```python
from build123d import *

# Parameters (mm, degrees)
SKETCH1_W           = 100
SKETCH1_H           = 300
SKETCH1_W_2         = 88
SKETCH1_H_2         = 91
SKETCH1_H_3         = 94
BOSS_EXTRUDE1_DEPTH = 6
SKETCH2_R           = 1.5
CUT_EXTRUDE1_DEPTH  = 6


with BuildPart() as part:
    # Sketch1 → Boss-Extrude1 (new body)
    with BuildSketch(Plane.XY):
        Rectangle(SKETCH1_W, SKETCH1_H)
        with Locations((0, 98.5)):
            Rectangle(SKETCH1_W_2, SKETCH1_H_2, mode=Mode.SUBTRACT)
        with Locations((0, -98.5)):
            Rectangle(SKETCH1_W_2, SKETCH1_H_2, mode=Mode.SUBTRACT)
        Rectangle(SKETCH1_W_2, SKETCH1_H_3, mode=Mode.SUBTRACT)
    extrude(amount=BOSS_EXTRUDE1_DEPTH)

    # Sketch2 → Cut-Extrude1 (cut)
    with BuildSketch(Plane.XY.offset(6)):
        with Locations((-47, 147)):
            Circle(SKETCH2_R)
        with Locations((47, 147)):
            Circle(SKETCH2_R)
        with Locations((47, 49)):
            Circle(SKETCH2_R)
        with Locations((47, -49)):
            Circle(SKETCH2_R)
        with Locations((47, -147)):
            Circle(SKETCH2_R)
        with Locations((-47, 49)):
            Circle(SKETCH2_R)
        with Locations((-47, -49)):
            Circle(SKETCH2_R)
        with Locations((-47, -147)):
            Circle(SKETCH2_R)
    extrude(amount=-CUT_EXTRUDE1_DEPTH, mode=Mode.SUBTRACT)


solid = part.part
```
CAD build for the part. Positions are in the model's coordinates, mm. A direction names the side the tool comes from. Round coordinates to 2 decimals unless told otherwise and drop trailing zeros. Write each loop counter-clockwise with the first axis right and the second up, starting at its lowest first coordinate (ties: lowest second). Pieces come first, ordered by that corner, then holes. Notation, with made-up numbers: (14.5, 77.25) - (24.5, 77.25) arc R21 cw to (24.5, 88.25) - close; hole circle Ø5 at (-4.5, 13.25). An arc over 180 degrees is marked (long way). Return JSON: item names as keys, results as strings. Group by question number.
Item 1: Band-saw the part on B-B on x = 1. List the corners of the cut face in (y, z).
Item 2: Probe probe 1 along Y at (x, z) = (-38, 3.9); probe 2 along Y at (x, z) = (47, 4.5); probe 3 along X at (y, z) = (147, 2.15). List the from-to ranges inside material, lowest first.
Item 3: Mould opens along X. For faces 3 (the face through (50, -2, 3)), 4 (the face through (-45, 23, 0)), 5 (the face through (44, -1, 3)) say: +X half, -X half, draft (parallel to the pull), parting line (faces both ways), or undercut.
Item 4: Band-saw the part on C-C on z = 4. State how many separate pieces and enclosed holes the cut face has, plus the area to 3 significant figures.
Item 5: 3-axis set-ups, long thin cutter, end or side, ignore diameter. For faces 1 (the face through (-1, -53, 3)), 2 (the face through (-1, 150, 3)): which of +Z, -Z, +X, -X, +Y, -Y reach the whole face in a straight line?
Item 6: Flat gauge pin, fed straight in: pin 1 Ø1.8 at (x, y) = (47, -49) entering from -Z. Where does the tip first touch, or does it go through?
Item 7: Band-saw the part on A-A on y = 80.5. List the corners of the cut face in (x, z), plus the area to 3 significant figures.
Resolved:
{
 "1": {"outline": "(-150, 0) - (-144, 0) - (-144, 6) - (-150, 6) - close; (-53, 0) - (-47, 0) - (-47, 6) - (-53, 6) - close; (47, 0) - (53, 0) - (53, 6) - (47, 6) - close; (144, 0) - (150, 0) - (150, 6) - (144, 6) - close"},
 "2": {"probe 1": "y = -150 to -144, -53 to -47, 47 to 53, 144 to 150", "probe 2": "y = -150 to -148.5, -145.5 to -50.5, -47.5 to 47.5, 50.5 to 145.5, 148.5 to 150", "probe 3": "x = -50 to -48.5, -45.5 to 45.5, 48.5 to 50"},
 "3": {"face 3": "+X half", "face 4": "draft", "face 5": "undercut"},
 "4": {"separate pieces": "1", "enclosed holes": "11", "area": "5,660 mm²"},
 "5": {"face 1": "+Z, -Z", "face 2": "+Z, -Z, +X, -X, +Y"},
 "6": {"pin 1": "passes through"},
 "7": {"outline": "(-50, 0) - (-44, 0) - (-44, 6) - (-50, 6) - close; (44, 0) - (50, 0) - (50, 6) - (44, 6) - close", "area": "72.0 mm²"}
}
